from build123d import *

# Parameters (mm, degrees)
SKETCH1_R           = 18
SKETCH1_R_2         = 11.5
SKETCH1_R_3         = 1.525
BOSS_EXTRUDE1_DEPTH = 0.79375


with BuildPart() as part:
    # Sketch1 → Boss-Extrude1 (new body)
    with BuildSketch(Plane.XY):
        Circle(SKETCH1_R)
        Circle(SKETCH1_R_2, mode=Mode.SUBTRACT)
        with Locations((0, 14.5)):
            Circle(SKETCH1_R_3, mode=Mode.SUBTRACT)
        with Locations((13.790319486, 4.480746418)):
            Circle(SKETCH1_R_3, mode=Mode.SUBTRACT)
        with Locations((8.522886158, -11.730746418)):
            Circle(SKETCH1_R_3, mode=Mode.SUBTRACT)
        with Locations((-8.522886158, -11.730746418)):
            Circle(SKETCH1_R_3, mode=Mode.SUBTRACT)
        with Locations((-13.790319486, 4.480746418)):
            Circle(SKETCH1_R_3, mode=Mode.SUBTRACT)
    extrude(amount=BOSS_EXTRUDE1_DEPTH)


solid = part.part
Can you work these out from the model? Positions are in its coordinate system, mm. Round coordinates to 2 decimals unless told otherwise and drop trailing zeros. Loops run counter-clockwise (first coordinate to the right, second up) from the corner with the lowest first, then second, coordinate; pieces in that order, holes last. Notation, with made-up numbers: (-16, -4.75) - (10, -4.75) arc R22 cw to (10, 29.25) - close; hole circle Ø6 at (-34.75, -18.5). An arc over 180 degrees is marked (long way). Answer in a Markdown table with one row per item. Add a question column.
Q1. I want a section at B-B on x = 0. List the corners of the cut face in (y, z) for me (3 decimals).
Q2. For pin 1 Ø2.5 at (x, y) = (-13.79, 4.48) entering from +Z, with a flat end and sliding along its axis, tell me the tip position at first contact or that it passes through.
Q3. I want a section at D-D on y = 14.5. List the corners of the cut face in (x, z) for me (3 decimals), and give its area (3 significant figures).
Q4. I want a section at C-C on z = 0.6. List the corners of the cut face in (x, y) for me (3 decimals), and give its area (3 significant figures).
Q5. I want a section at A-A on y = 0. List the corners of the cut face in (x, z) for me.
Q6. We'd pull the mould along Y, two halves only. Please class faces 1 (the flat face through (12, 0, 0)), 2 (the cylindrical face through (-2.343, 17.847, 0.391)), 3 (the cylindrical face through (-0.33, 13.01, 0.39)): pulls with the +Y half, pulls with the -Y half, needs draft (parallel to the pull), parting line crosses it, or undercut.
Q7. I need wall thicknesses on L1, parallel to Y at x = 0, z = 0.2 (3 decimals); L2, parallel to Y at x = -8.5, z = 0.35; L3, parallel to X at y = 5.5, z = 0.05. Which ranges of each line are inside material? Lowest first, please.
A:
| question | item | result |
|---|---|---|
| 1 | outline | (-18, 0) - (-11.5, 0) - (-11.5, 0.794) - (-18, 0.794) - close; (11.5, 0) - (12.975, 0) - (12.975, 0.794) - (11.5, 0.794) - close; (16.025, 0) - (18, 0) - (18, 0.794) - (16.025, 0.794) - close |
| 2 | pin 1 | through |
| 3 | outline | (-10.665, 0) - (-1.525, 0) - (-1.525, 0.794) - (-10.665, 0.794) - close; (1.525, 0) - (10.665, 0) - (10.665, 0.794) - (1.525, 0.794) - close |
| 3 | area | 14.5 mm^2 |
| 4 | outline | circle Ø36 at (0, 0); hole circle Ø3.05 at (-13.79, 4.481); hole circle Ø23 at (0, 0); hole circle Ø3.05 at (-8.523, -11.731); hole circle Ø3.05 at (0, 14.5); hole circle Ø3.05 at (8.523, -11.731); hole circle Ø3.05 at (13.79, 4.481) |
| 4 | area | 566 mm^2 |
| 5 | outline | (-18, 0) - (-11.5, 0) - (-11.5, 0.79) - (-18, 0.79) - close; (11.5, 0) - (18, 0) - (18, 0.79) - (11.5, 0.79) - close |
| 6 | face 1 | needs draft |
| 6 | face 2 | parting line crosses it |
| 6 | face 3 | undercut |
| 7 | L1 | -18 to -11.5, 11.5 to 12.975, 16.025 to 18 |
| 7 | L2 | -15.87 to -13.26, -10.21 to -7.75, 7.75 to 15.87 |
| 7 | L3 | -17.14 to -14.92, -12.66 to -10.1, 10.1 to 12.66, 14.92 to 17.14 |
